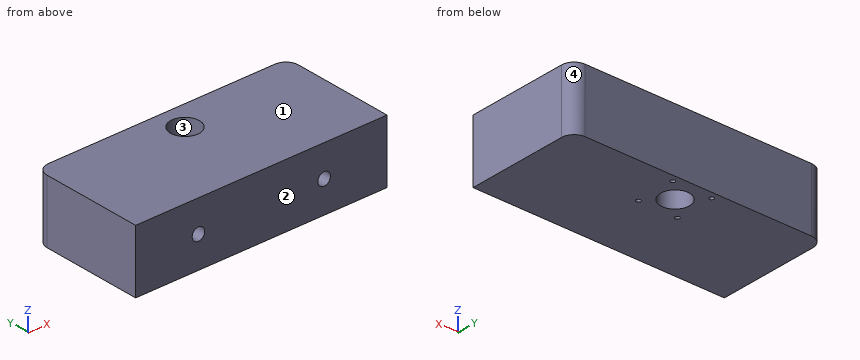
from build123d import *

# Parameters (mm, degrees)
SKETCH1_W           = 200
SKETCH1_H           = 90
SKETCH1_R           = 11.5
BOSS_EXTRUDE1_DEPTH = 25
SKETCH2_R           = 1.75
CUT_EXTRUDE1_DEPTH  = 10
SKETCH3_R           = 5
CUT_EXTRUDE2_DEPTH  = 15
FILLET1_R           = 10


with BuildPart() as part:
    # Sketch1 → Boss-Extrude1 (new body, symmetric)
    with BuildSketch(Plane.XY):
        Rectangle(SKETCH1_W, SKETCH1_H)
        with Locations((0, 24)):
            Circle(SKETCH1_R, mode=Mode.SUBTRACT)
    extrude(amount=BOSS_EXTRUDE1_DEPTH, both=True)

    # Sketch2 → Cut-Extrude1 (cut)
    with BuildSketch(Plane(origin=(0, 0, -25), x_dir=(-1, 0, 0), z_dir=(0, 0, -1))):
        with Locations((-15.5, 8.5)):
            Circle(SKETCH2_R)
        with Locations((15.5, 8.5)):
            Circle(SKETCH2_R)
        with Locations((15.5, 39.5)):
            Circle(SKETCH2_R)
        with Locations((-15.5, 39.5)):
            Circle(SKETCH2_R)
    extrude(amount=-CUT_EXTRUDE1_DEPTH, mode=Mode.SUBTRACT)

    # Sketch3 → Cut-Extrude2 (cut)
    with BuildSketch(Plane.XZ.offset(45)):
        with Locations((-50, 0)):
            Circle(SKETCH3_R)
        with Locations((50, 0)):
            Circle(SKETCH3_R)
    extrude(amount=-CUT_EXTRUDE2_DEPTH, mode=Mode.SUBTRACT)

    # Fillet1
    fillet1_edges = [part.edges().sort_by_distance(p)[0] for p in [
        (100, 45, 0),
        (-100, 45, 0),
    ]]
    fillet(fillet1_edges, radius=FILLET1_R)


solid = part.part
Work out the finished part from the listing and answer in its coordinate system (mm). Face numbers are marked on the shaded views. Give positions to 0.01 mm unless a question says otherwise; leave off trailing zeros. Loops run counter-clockwise (first coordinate to the right, second up) from the corner with the lowest first, then second, coordinate; pieces in that order, holes last. Notation, with made-up numbers: (73, -0.5) - (97, -0.5) arc R20 cw to (97, 20.5) - close; hole circle Ø5 at (0, -39.5). An arc over 180 degrees is marked (long way). Answer in a Markdown table with one row per item.
(1) Consider L1, parallel to Y at x = -15.5, z = -21.75; L2, parallel to X at y = 25, z = 15; L3, parallel to Y at x = 0, z = 3. Determine where each line is inside the solid, lowest interval first. Write a range as [from, to].
Results list:
| item | result |
|---|---|
| L1 | y = [-45, 6.75], [10.25, 37.75], [41.25, 45] |
| L2 | x = [-100, -11.46], [11.46, 100] |
| L3 | y = [-45, 12.5], [35.5, 45] |
(2) Section D-D (y = -38) is taken. Give the vertices of the cut face in (x, z), and give its area (3 significant figures).
Results list:
| item | result |
|---|---|
| outline | (-100, -25) - (100, -25) - (100, 25) - (-100, 25) - close; hole circle Ø10 at (-50, 0); hole circle Ø10 at (50, 0) |
| area | 9,840 mm² |
(3) Section B-B (z = 0) is taken. Give the vertices of the cut face in (x, y), and give its area (3 significant figures).
Results list:
| item | result |
|---|---|
| outline | (-100, -45) - (-55, -45) - (-55, -30) - (-45, -30) - (-45, -45) - (45, -45) - (45, -30) - (55, -30) - (55, -45) - (100, -45) - (100, 35) arc R10 ccw to (90, 45) - (-90, 45) arc R10 ccw to (-100, 35) - close; hole circle Ø23 at (0, 24) |
| area | 17,200 mm² |
(4) Flat-ended cylindrical pins translate along their axes: pin 1 Ø4 at (x, y) = (-15.5, 9) entering from -Z; pin 2 Ø1 at (x, y) = (14.5, 39.5) entering from -Z. Find the tip coordinate at first contact, or state that the pin passes through.
Results list:
| item | result |
|---|---|
| pin 1 | stops at z = -25 |
| pin 2 | stops at z = -15 |
(5) For a pull along Y with two mould halves and no side action, classify the marked faces 1, 2, 3 and 4 as pulls with the +Y half, pulls with the -Y half, needs draft (parallel to the pull), parting line crosses it, or undercut.
Results list:
| item | result |
|---|---|
| face 1 | needs draft |
| face 2 | pulls with the -Y half |
| face 3 | undercut |
| face 4 | pulls with the +Y half |
(6) Section A-A (x = 0) is taken. Give the vertices of the cut face in (y, z).
Results list:
| item | result |
|---|---|
| outline | (-45, -25) - (12.5, -25) - (12.5, 25) - (-45, 25) - close; (35.5, -25) - (45, -25) - (45, 25) - (35.5, 25) - close |
(7) Section C-C (x = 50) is taken. Give the vertices of the cut face in (y, z).
Results list:
| item | result |
|---|---|
| outline | (-45, -25) - (45, -25) - (45, 25) - (-45, 25) - (-45, 5) - (-30, 5) - (-30, -5) - (-45, -5) - close |
